Verification items for the finished model (mm, model axes). A direction names the side the tool comes from. Coordinates: 2 decimals unless noted, no trailing zeros. Write each loop counter-clockwise with the first axis right and the second up, starting at its lowest first coordinate (ties: lowest second). Pieces come first, ordered by that corner, then holes. Notation, with made-up numbers: M 28.25,-26 L 45.25,-26 A22 ccw 45.25,12 Z; hole C 28.25,28 d10. An arc over 180 degrees is marked long. Answer in a Markdown table with one row per item.
from build123d import *

# Parameters (mm, degrees)
F1_R     = 14.31925
F1_W     = 12.7
F1_H     = 3.175
F1_W_2   = 6.604
F1_H_2   = 12.7
F2_DEPTH = 6.604


with BuildPart() as f2:
    # F1 (on offset) → F2 (new body)
    with BuildSketch(Plane.YZ.offset(101.6)):
        Polygon((28.575, 0), (28.575, 69.85), (0, 69.85), (-28.575, 69.85), (-28.575, 58.7375), (-28.575, 46.0375), (-28.575, 23.8125), (-28.575, 11.1125), (-28.575, 0), (-20.6375, 0), (-7.9375, 0), (7.9375, 0), (20.6375, 0), align=None)
        with BuildLine():
            Line((0, 69.85), (28.575, 69.85))
            Line((28.575, 69.85), (28.575, 98.425))
            ThreePointArc((28.575, 98.425), (20.205576, 78.219424), (0, 69.85))
        make_face()
        with BuildLine():
            Line((-28.575, 69.85), (0, 69.85))
            ThreePointArc((0, 69.85), (-20.205576, 78.219424), (-28.575, 98.425))
            Line((-28.575, 98.425), (-28.575, 69.85))
        make_face()
        with BuildLine():
            ThreePointArc((-28.575, 98.425), (-20.205576, 78.219424), (0, 69.85))
            ThreePointArc((0, 69.85), (20.205576, 78.219424), (28.575, 98.425))
            ThreePointArc((28.575, 98.425), (0, 127), (-28.575, 98.425))
        make_face()
        with Locations((0, 98.425)):
            Circle(F1_R, mode=Mode.SUBTRACT)
        with Locations((14.2875, -1.5875)):
            Rectangle(F1_W, F1_H)
        with Locations((-31.877, 52.3875)):
            Rectangle(F1_W_2, F1_H_2)
        with Locations((-14.2875, -1.5875)):
            Rectangle(F1_W, F1_H)
        with Locations((-31.877, 17.4625)):
            Rectangle(F1_W_2, F1_H_2)
    extrude(amount=F2_DEPTH)


solid = f2.part
1) Release check for a two-part mould opening along Z. For faces 5 (the face through (105, -32, 23.812)), 6 (the face through (105, -25, 0)), 7 (the face through (105, -20.638, -2)) record: +Z half, -Z half, draft (parallel to the pull), parting line (faces both ways), or undercut.
Response values:
| item | result |
|---|---|
| face 5 | undercut |
| face 6 | -Z half |
| face 7 | draft |
2) Sectioned sample at D-D (y = -24). Record the cut outline in (x, z), then the cut area to 3 significant figures.
Response values:
| item | result |
|---|---|
| outline | M 101.6,0 L 108.2,0 L 108.2,113.93 L 101.6,113.93 Z |
| area | 752 mm² |
3) Sectioned sample at C-C (z = 27.5). Record the cut outline in (x, y) (3 decimals), then the cut area to 3 significant figures.
Response values:
| item | result |
|---|---|
| outline | M 101.6,-28.575 L 108.204,-28.575 L 108.204,28.575 L 101.6,28.575 Z |
| area | 377 mm² |
4) Thickness scan on L1, parallel to Z at x = 104, y = 0; L2, parallel to Y at x = 102.5, z = 41 (3 decimals); L3, parallel to Y at x = 104.75, z = 109. Record the ranges inside material, lowest first. Write a range as [from, to].
Response values:
| item | result |
|---|---|
| L1 | z = [0, 84.11], [112.74, 127] |
| L2 | y = [-28.575, 28.575] |
| L3 | y = [-26.55, -9.65], [9.65, 26.55] |
5) Depth check by flat-ended pin: pin 1 (3.5 mm diameter, centred on x = 105.5, y = -33, fed in from +Z); pin 2 (2 mm diameter, centred on x = 103.5, y = 23, fed in from -Z); pin 3 (2.5 mm diameter, centred on x = 105.5, z = -1, fed in from -Y) (3 decimals). Enter the tip coordinate at first touch or a pass-through.
Response values:
| item | result |
|---|---|
| pin 1 | stops at z = 58.74 |
| pin 2 | stops at z = 0 |
| pin 3 | stops at y = -28.575 |
6) Tool access check on faces 1 (the face through (105, 0, 0)), 2 (the face through (105, -28.575, 79)), 3 (the face through (105, 20.638, -2)), 4 (the face through (105, -28.575, 35)). Record the directions out of +Z, -Z, +X, -X, +Y, -Y that give a thin tool (end or side, any length) a straight path to the whole face; none if there is none.
Response values:
| item | result |
|---|---|
| face 1 | -Z, +X, -X |
| face 2 | +Z, +X, -X, -Y |
| face 3 | -Z, +X, -X, +Y |
| face 4 | +X, -X, -Y |
7) Sectioned sample at A-A (y = -1.5). Record the cut outline in (x, z).
Response values:
| item | result |
|---|---|
| outline | M 101.6,0 L 108.2,0 L 108.2,84.18 L 101.6,84.18 Z; M 101.6,112.67 L 108.2,112.67 L 108.2,126.96 L 101.6,126.96 Z |
